```python
from build123d import *

# Parameters (mm, degrees)
BOSS_EXTRUDE1_DEPTH          = 16
F_6_0_6_DIAMETER_HOLE1_D     = 6
F_6_0_6_DIAMETER_HOLE1_DEPTH = 6


with BuildPart() as part:
    # Sketch1 → Boss-Extrude1 (new body)
    with BuildSketch(Plane(origin=(8, 0, 0), x_dir=(0, 0, -1), z_dir=(1, 0, 0))):
        Polygon((-0.2, 0), (-4, 0), (-4, -2), (-8.25, -2), (-8.25, -3), (-5.25, -6), (5.25, -6), (8.25, -3), (8.25, -2), (4, -2), (4, 0), (0.2, 0), (0, -0.2), align=None)
    extrude(amount=-BOSS_EXTRUDE1_DEPTH)

    # Ø6.0 (6) Diameter Hole1
    with Locations(Plane.XZ.offset(6)):
        with Locations((0, 0)):
            Hole(F_6_0_6_DIAMETER_HOLE1_D / 2, depth=F_6_0_6_DIAMETER_HOLE1_DEPTH)


solid = part.part
```
Work out the finished part from the listing and answer in its coordinate system (mm). A direction names the side the tool comes from. Coordinates: 2 decimals unless noted, no trailing zeros. Write each loop counter-clockwise with the first axis right and the second up, starting at its lowest first coordinate (ties: lowest second). Pieces come first, ordered by that corner, then holes.
Q1. Which of the six approach directions +Z, -Z, +X, -X, +Y, -Y give full straight-line access (tool end or side, diameter ignored) to faces 4 (the face through (8, -3, 0)), 5 (the face through (0, -2, 6)), 6 (the face through (0, -1, -4))?
Q2. Each of these flat-tipped pins is pushed along its axis until it touches: pin 1 Ø5.5 at (x, z) = (0, 0) entering from +Y; pin 2 Ø3.5 at (x, z) = (-3, -7) entering from +Y; pin 3 Ø2 at (x, y) = (0.5, -0.5) entering from -Z; pin 4 Ø5 at (x, z) = (0.5, -3) entering from +Y. Where does it stop, or does it pass through?
Q3. A cutting plane is placed at A-A, the plane x = 0. Give the vertices of the cut face in (y, z).
Q4. A cutting plane is placed at D-D, the plane z = -6.5. Give the vertices of the cut face in (x, y), then the cut area to 3 significant figures.
Q5. A cutting plane is placed at B-B, the plane y = -0.5. Give the vertices of the cut face in (x, z), then the cut area to 3 significant figures.
Q6. A cutting plane is placed at C-C, the plane x = -6. Give the vertices of the cut face in (y, z).
Q7. Determine the mould class of faces 1 (the face through (3, -3, 0)), 2 (the face through (0.1, -2.5, -8.25)), 3 (the face through (-8, -3, 0)) for opening direction Z: released by +Z, released by -Z, zero draft, split by the parting line, or undercut.
Q8. Find the intervals of material crossed by line 1 (X direction, y = -1, z = 0); line 2 (Z direction, x = 0, y = -1.25); line 3 (Z direction, x = 0, y = -2.5), in increasing order.
Findings below:
1. face 4: +Z, -Z, +X, +Y, -Y
1. face 5: +Z, +X, -X, +Y
1. face 6: -Z, +X, -X, +Y
2. pin 1: passes through
2. pin 2: stops at y = -2
2. pin 3: stops at z = -4
2. pin 4: stops at y = 0
3. outline: (-6, -5.25) - (-3, -8.25) - (-2, -8.25) - (-2, -4) - (0, -4) - (0, -3) - (-6, -3) - close; (-6, 3) - (0, 3) - (0, 4) - (-2, 4) - (-2, 8.25) - (-3, 8.25) - (-6, 5.25) - close
4. outline: (-8, -4.75) - (8, -4.75) - (8, -2) - (-8, -2) - close
4. area: 44.0 mm2
5. outline: (-8, -4) - (8, -4) - (8, 4) - (-8, 4) - close; hole circle Ø6 at (0, 0)
5. area: 99.7 mm2
6. outline: (-6, -5.25) - (-3, -8.25) - (-2, -8.25) - (-2, -4) - (0, -4) - (0, -0.2) - (-0.2, 0) - (0, 0.2) - (0, 4) - (-2, 4) - (-2, 8.25) - (-3, 8.25) - (-6, 5.25) - close
7. face 1: undercut
7. face 2: released by -Z
7. face 3: zero draft
8. line 1: x = -8 to -3, 3 to 8
8. line 2: z = -4 to -3, 3 to 4
8. line 3: z = -8.25 to -3, 3 to 8.25
